The listing builds one solid part. Answer for the finished solid, in the listing's coordinates (mm). Round coordinates to 2 decimals unless told otherwise and drop trailing zeros. Loops run counter-clockwise (first coordinate to the right, second up) from the corner with the lowest first, then second, coordinate; pieces in that order, holes last. Notation, with made-up numbers: (22, -35) - (78, -35) arc R28 ccw to (78, 3) - close; hole circle Ø1 at (-24.75, 11). An arc over 180 degrees is marked (long way). One line per item, written item: value.
```python
from build123d import *

# Parameters (mm, degrees)
F1_DEPTH = 5
F2_SIZE  = 1


with BuildPart() as f1:
    # F0 (on Front) → F1 (new body)
    with BuildSketch(Plane.XZ):
        with BuildLine():
            Line((79.487856, 150.528029), (-20.512144, 150.528029))
            Line((-20.512144, 150.528029), (-20.512144, 3.028029))
            Line((-20.512144, 3.028029), (9.487856, 3.028029))
            ThreePointArc((9.487856, 3.028029), (11.987856, 0.528029), (9.487856, -1.971971))
            Line((9.487856, -1.971971), (-20.512144, -1.971971))
            Line((-20.512144, -1.971971), (-20.512144, -49.471971))
            Line((-20.512144, -49.471971), (79.487856, -49.471971))
            Line((79.487856, -49.471971), (79.487856, -1.971971))
            Line((79.487856, -1.971971), (49.487856, -1.971971))
            ThreePointArc((49.487856, -1.971971), (46.987856, 0.528029), (49.487856, 3.028029))
            Line((49.487856, 3.028029), (79.487856, 3.028029))
            Line((79.487856, 3.028029), (79.487856, 150.528029))
        make_face()
    extrude(amount=F1_DEPTH)

    # F2
    f2_edges = [f1.edges().sort_by_distance(p)[0] for p in [
        (29.487856, -5, 150.528029),
        (-20.512144, -5, 76.778029),
        (-5.512144, -5, 3.028029),
        (11.987856, -5, 0.528029),
        (-5.512144, -5, -1.971971),
        (-20.512144, -5, -25.721971),
        (29.487856, -5, -49.471971),
        (79.487856, -5, -25.721971),
        (64.487856, -5, -1.971971),
        (46.987856, -5, 0.528029),
        (64.487856, -5, 3.028029),
        (79.487856, -5, 76.778029),
        (29.487856, 0, 150.528029),
        (-20.512144, 0, 76.778029),
        (-5.512144, 0, 3.028029),
        (11.987856, 0, 0.528029),
        (-5.512144, 0, -1.971971),
        (-20.512144, 0, -25.721971),
        (29.487856, 0, -49.471971),
        (79.487856, 0, -25.721971),
        (64.487856, 0, -1.971971),
        (46.987856, 0, 0.528029),
        (64.487856, 0, 3.028029),
        (79.487856, 0, 76.778029),
        (-20.512144, -2.5, -49.471971),
        (79.487856, -2.5, -49.471971),
        (79.487856, -2.5, 150.528029),
        (-20.512144, -2.5, 150.528029),
    ]]
    chamfer(f2_edges, length=F2_SIZE)


solid = f1.part
```
1) A cutting plane is placed at A-A on x = -5.5. Give the vertices of the cut face in (y, z), and give its area (3 significant figures).
Final values:
outline: (-5, -48.47) - (-4, -49.47) - (-1, -49.47) - (0, -48.47) - (0, -2.97) - (-1, -1.97) - (-4, -1.97) - (-5, -2.97) - close; (-5, 4.03) - (-4, 3.03) - (-1, 3.03) - (0, 4.03) - (0, 149.53) - (-1, 150.53) - (-4, 150.53) - (-5, 149.53) - close
area: 971 mm2
2) For a pull along Z with two mould halves and no side action, classify faces 1 (the conical face through (46.815, -4.174, 0.469)), 2 (the conical face through (12.161, -4.174, 0.587)), 3 (the flat face through (29, -5, 52)) as released by +Z, released by -Z, zero draft, split by the parting line, or undercut.
Final values:
face 1: undercut
face 2: undercut
face 3: zero draft
3) Consider L1, parallel to Z at x = -12.5, y = -1.9; L2, parallel to Z at x = -11, y = -4.55; L3, parallel to X at y = -4.15, z = 79. Determine where each line is inside the solid, lowest interval first.
Final values:
L1: -49.47 to -1.97, 3.03 to 150.53
L2: -48.92 to -2.52, 3.58 to 149.98
L3: -20.36 to 79.34
4) A cutting plane is placed at B-B on y = -2.25. Give the vertices of the cut face in (x, z), and give its area (3 significant figures).
Final values:
outline: (-20.51, -48.47) - (-19.51, -49.47) - (78.49, -49.47) - (79.49, -48.47) - (79.49, -1.97) - (49.49, -1.97) arc R2.5 cw to (49.49, 3.03) - (79.49, 3.03) - (79.49, 149.53) - (78.49, 150.53) - (-19.51, 150.53) - (-20.51, 149.53) - (-20.51, 3.03) - (9.49, 3.03) arc R2.5 cw to (9.49, -1.97) - (-20.51, -1.97) - close
area: 19,700 mm2
